Answer from the drawing. Dimensions are ordinates in mm from the lowest x, y and z of the part. A direction names the side the tool comes from. Round coordinates to 2 decimals unless told otherwise and drop trailing zeros. Write each loop counter-clockwise with the first axis right and the second up, starting at its lowest first coordinate (ties: lowest second). Pieces come first, ordered by that corner, then holes. Notation, with made-up numbers: M -21,31 L 19,31 A27 cw 19,48 Z; hole C 44,7.25 d5. An arc over 180 degrees is marked long. Answer as CSV lines item,"result". Start each with the question number.
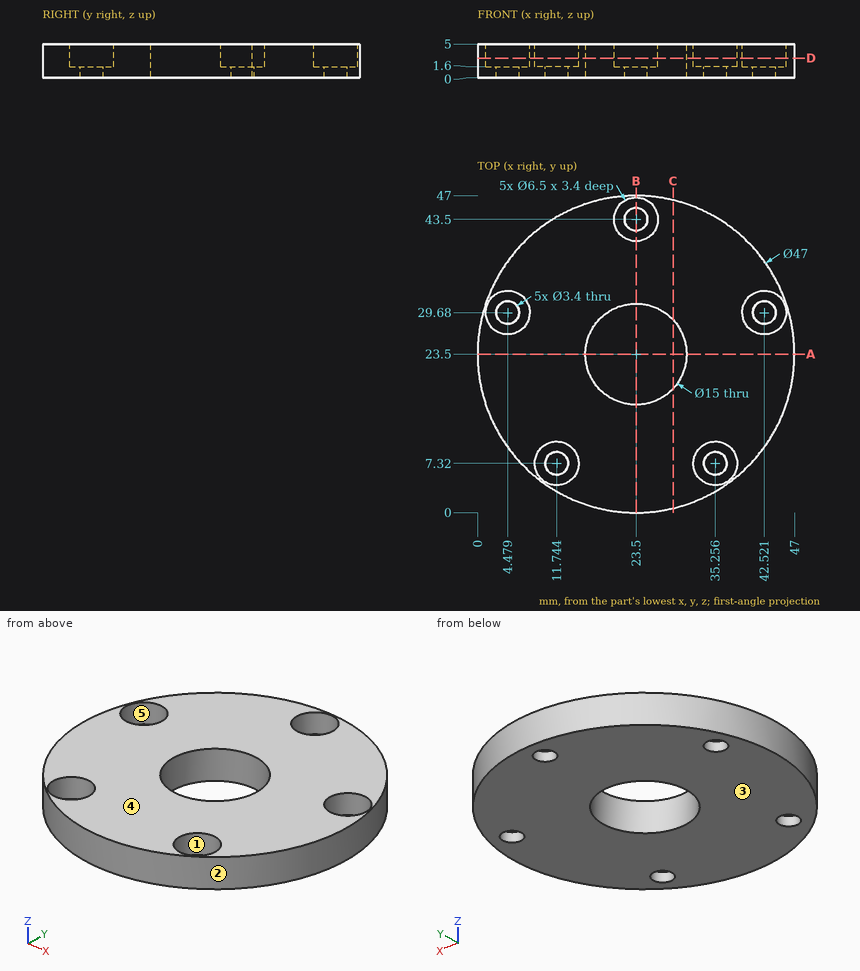
Q1. For the marked faces 4 and 5, determine the directions among +Z, -Z, +X, -X, +Y, -Y from which every point of the face is accessible in a straight line to the end or side of a thin tool.
Q2. Find section A-A (y = 23.5). Determine the outline of the cut face in (x, z).
Q3. Find section C-C (x = 29). Determine the outline of the cut face in (y, z).
Q4. Find section D-D (z = 2.9). Count the separate pieces of the cut face and the enclosed holes in it, plus the area to 3 significant figures.
Q5. The mould has two halves that part along Y. Classify the marked faces 1, 2 and 3: +Y half, -Y half, draft (parallel to the pull), parting line (faces both ways), or undercut.
Q6. Find section B-B (x = 23.5). Determine the outline of the cut face in (y, z).
Q7. Straight lines are drawn through the part: L1, parallel to Y at x = 23.5, z = 3.45; L2, parallel to X at y = 27.5, z = 3.25 (1 decimal); L3, parallel to X at y = 18, z = 3.3. For each, find the intervals that lie inside material, in ascending order.
Q8. Each of these flat-tipped pins is pushed along its axis until it touches: P1, Ø3, axis at x = 24.5, y = 40, coming from the -Z side; P2, Ø3, axis at x = 6, z = 3, coming from the -Y side; P3, Ø5.5, axis at x = 4.48, y = 29.68, coming from the +Z side; P4, Ø3, axis at x = 15.5, z = 3.5, coming from the -Y side. Where does it stop, or does it pass through?
Reported:
1,face 4,"+Z, +X, -X, +Y, -Y"
1,face 5,"+Z"
2,outline,"M 0,0 L 16,0 L 16,5 L 0,5 Z; M 31,0 L 47,0 L 47,5 L 31,5 Z"
3,outline,"M 0.65,0 L 18.4,0 L 18.4,5 L 0.65,5 Z; M 28.6,0 L 46.35,0 L 46.35,5 L 28.6,5 Z"
4,separate pieces,"1"
4,enclosed holes,"6"
4,area,"1,390 mm2"
5,face 1,"undercut"
5,face 2,"parting line"
5,face 3,"draft"
6,outline,"M 0,0 L 16,0 L 16,5 L 0,5 Z; M 31,0 L 41.8,0 L 41.8,1.6 L 40.25,1.6 L 40.25,5 L 31,5 Z; M 45.2,0 L 47,0 L 47,5 L 46.75,5 L 46.75,1.6 L 45.2,1.6 Z"
7,L1,"y = 0 to 16, 31 to 40.25, 46.75 to 47"
7,L2,"x = 0.3 to 2.1, 6.9 to 17.2, 29.8 to 40.1, 44.9 to 46.7"
7,L3,"x = 0.65 to 18.4, 28.6 to 46.35"
8,P1,"stops at z = 0"
8,P2,"stops at y = 6.29"
8,P3,"stops at z = 1.6"
8,P4,"stops at y = 0.92"
